```python
from build123d import *

# Parameters (mm, degrees)
SKETCH_1_R             = 2
SM_BASE_FLANGE_1_DEPTH = 2


# Sheet-metal steps are written as plain solids
with BuildPart() as part:
    # Sketch 1 → 基体-法兰1 (new body)
    with BuildSketch(Plane(origin=(0, 0, 0), x_dir=(1, 0, 0), z_dir=(0, 1, 0))):
        with BuildLine():
            Line((-165, 225), (165, 225))
            ThreePointArc((165, 225), (172.071067812, 222.071067812), (175, 215))
            Line((175, 215), (175, -215))
            ThreePointArc((175, -215), (172.071067812, -222.071067812), (165, -225))
            Line((165, -225), (-165, -225))
            ThreePointArc((-165, -225), (-172.071067812, -222.071067812), (-175, -215))
            Line((-175, -215), (-175, 215))
            ThreePointArc((-175, 215), (-172.071067812, 222.071067812), (-165, 225))
        make_face()
        with Locations(Location((-165, 190, 0), (0, 0, 270))):
            Circle(SKETCH_1_R, mode=Mode.SUBTRACT)
        with Locations(Location((165, 190, 0), (0, 0, 270))):
            Circle(SKETCH_1_R, mode=Mode.SUBTRACT)
        with Locations(Location((165, 0, 0), (0, 0, 270))):
            Circle(SKETCH_1_R, mode=Mode.SUBTRACT)
        with Locations(Location((165, -190, 0), (0, 0, 270))):
            Circle(SKETCH_1_R, mode=Mode.SUBTRACT)
        with Locations(Location((-165, -190, 0), (0, 0, 270))):
            Circle(SKETCH_1_R, mode=Mode.SUBTRACT)
        with Locations(Location((-165, 0, 0), (0, 0, 270))):
            Circle(SKETCH_1_R, mode=Mode.SUBTRACT)
        with BuildLine():
            Line((-158.5, 137), (-138.5, 137))
            ThreePointArc((-138.5, 137), (-136.5, 135), (-138.5, 133))
            Line((-138.5, 133), (-158.5, 133))
            ThreePointArc((-158.5, 133), (-160.5, 135), (-158.5, 137))
        make_face(mode=Mode.SUBTRACT)
        with BuildLine():
            Line((138.5, 137), (158.5, 137))
            ThreePointArc((158.5, 137), (160.5, 135), (158.5, 133))
            Line((158.5, 133), (138.5, 133))
            ThreePointArc((138.5, 133), (136.5, 135), (138.5, 137))
        make_face(mode=Mode.SUBTRACT)
        with BuildLine():
            Line((-158.5, -137), (-138.5, -137))
            ThreePointArc((-138.5, -137), (-136.5, -135), (-138.5, -133))
            Line((-138.5, -133), (-158.5, -133))
            ThreePointArc((-158.5, -133), (-160.5, -135), (-158.5, -137))
        make_face(mode=Mode.SUBTRACT)
        with BuildLine():
            Line((138.5, -137), (158.5, -137))
            ThreePointArc((158.5, -137), (160.5, -135), (158.5, -133))
            Line((158.5, -133), (138.5, -133))
            ThreePointArc((138.5, -133), (136.5, -135), (138.5, -137))
        make_face(mode=Mode.SUBTRACT)
    extrude(amount=-SM_BASE_FLANGE_1_DEPTH)


solid = part.part
```
Could you check a few things on this model? Use its own coordinates, in mm. Coordinates: 2 decimals unless noted, no trailing zeros. Use one line per item in the form item = value. Start each with the question number.
1. Please list where these lines run through material, in increasing order: line 1 (Z direction, x = 165, y = -1.3); line 2 (X direction, y = -0.55, z = 190); line 3 (Z direction, x = 159, y = -0.45).
2. For pin 1 (2.5 mm diameter, centred on x = 165, z = 190, fed in from +Y), with a flat end and sliding along its axis, tell me the tip position at first contact or that it passes through.
3. We'd pull the mould along X, two halves only. Please class faces 1 (the flat face through (2, 0, -3)), 2 (the cylindrical face through (172.15, -0.99, 221.99)), 3 (the cylindrical face through (-172.15, -0.99, -221.99)): +X half, -X half, draft (parallel to the pull), parting line (faces both ways), or undercut.
Geometry says:
q1.line_1 = -225 to -192, -188 to -2, 2 to 188, 192 to 225
q1.line_2 = -175 to -167, -163 to 163, 167 to 175
q1.line_3 = -225 to -136.94, -133.06 to 133.06, 136.94 to 225
q2.pin_1 = through
q3.face_1 = draft
q3.face_2 = +X half
q3.face_3 = -X half
